from build123d import *

# Parameters (mm, degrees)
BOSS_EXTRUDE1_DEPTH                               = 12.7
FILLET1_R                                         = 12.7
F_1_4_0_25_DIAMETER_HOLE1_D                       = 6.35
HOLE1_D                                           = 3.175
HOLE1_DEPTH                                       = 38.1
HOLE1_CSINK_D                                     = 10.16
HOLE1_CSINK_ANGLE                                 = 82
HOLE1_TIP                                         = 0.9538662327062519
F_5_16_CLEARANCE_HOLE1_D                          = 8.72998
CUT_EXTRUDE1_DEPTH                                = 998.2767957894854
FILLET2_R                                         = 3.175
CSK_FOR_8_FLAT_HEAD_MACHINE_SCREW_100_D           = 4.9149
CSK_FOR_8_FLAT_HEAD_MACHINE_SCREW_100_DEPTH       = 22.225
CSK_FOR_8_FLAT_HEAD_MACHINE_SCREW_100_CSINK_D     = 16.0004506
CSK_FOR_8_FLAT_HEAD_MACHINE_SCREW_100_CSINK_ANGLE = 100
CSK_FOR_8_FLAT_HEAD_MACHINE_SCREW_100_TIP         = 1.476584928229278


with BuildPart() as part:
    # Sketch1 → Boss-Extrude1 (new body)
    with BuildSketch(Plane.XY):
        Polygon((-504.586893891522, 825.1654748045078), (-413.82187552728277, 548.4721148571872), (-471.5394528912339, 529.5387477161187), (-562.3044712554732, 806.2321076634394), align=None)
        Polygon((-421.80123191535296, 572.7968488683923), (-413.82187552728277, 548.4721148571872), (-401.754552912923, 552.4306151945574), (-409.7339093009929, 576.7553492057625), align=None)
        Polygon((-504.586893891522, 825.1654748045078), (-492.51957127716224, 829.123975141878), (-484.5402148890918, 804.7992411306724), (-496.6075375034517, 800.8407407933022), align=None)
    extrude(amount=BOSS_EXTRUDE1_DEPTH)

    # Fillet1
    fillet1_edges = [part.edges().sort_by_distance(p)[0] for p in [
        (-401.754552912923, 552.4306151945574, 6.35),
        (-471.5394528912339, 529.5387477161187, 6.35),
        (-562.3044712554732, 806.2321076634394, 6.35),
        (-492.51957127716224, 829.123975141878, 6.35),
    ]]
    fillet(fillet1_edges, radius=FILLET1_R)

    # 1/4 (0.25) Diameter Hole1 (through all)
    with Locations(Plane(origin=(0, 0, 0), x_dir=(-1, 0, 0), z_dir=(0, 0, -1))):
        with Locations((496.607537503, 800.840740793), (421.801231915, 572.796848868)):
            Hole(F_1_4_0_25_DIAMETER_HOLE1_D / 2)

    # Hole1
    with Locations(Plane(origin=(-72.82198225638447, -450.30656055117834, -91.0749999969487), x_dir=(-4.8e-16, -1.6e-16, -1), z_dir=(0.9501828830204595, 0.3116929399504066, 0))):
        with Locations((-97.424999997, 1099.959715498), (-97.424999997, 1301.859715498), (-97.424999997, 1200.909715498)):
            CounterSinkHole(HOLE1_D / 2, HOLE1_CSINK_D / 2, depth=HOLE1_DEPTH, counter_sink_angle=HOLE1_CSINK_ANGLE)
            with Locations((0, 0, -(HOLE1_DEPTH + HOLE1_TIP / 2))):  # 118° drill point
                Cone(0, HOLE1_D / 2, HOLE1_TIP, mode=Mode.SUBTRACT)

    # 5/16 Clearance Hole1 (through all)
    with Locations(Plane.XY.offset(12.7)):
        with Locations((-546.278648304, 798.123285386), (-500.628393554, 813.09815219), (-463.430630614, 545.564570668), (-417.780375865, 560.539437472), (-501.837808805, 672.833553111)):
            Hole(F_5_16_CLEARANCE_HOLE1_D / 2)

    # Sketch9 → Cut-Extrude1 (cut, through all)
    with BuildSketch(Plane.XY.offset(12.7)):
        with BuildLine():
            Line((-529.6953014924577, 821.9412393048426), (-514.6111482245083, 826.8893647265553))
            ThreePointArc((-514.6111482245083, 826.8893647265553), (-508.60146461760905, 823.8485563726845), (-511.6422729714802, 817.838872765785))
            Line((-511.6422729714802, 817.838872765785), (-526.72642623943, 812.8907473440726))
            ThreePointArc((-526.72642623943, 812.8907473440726), (-532.7361098463288, 815.9315556979438), (-529.6953014924577, 821.9412393048426))
        make_face()
        with BuildLine():
            Line((-546.3745591048678, 778.043051296225), (-518.8053014409139, 693.9993230871839))
            ThreePointArc((-518.8053014409139, 693.9993230871839), (-522.8597125794092, 685.9864116113188), (-530.8726240552741, 690.0408227498137))
            Line((-530.8726240552741, 690.0408227498137), (-558.4418817192275, 774.084550958855))
            ThreePointArc((-558.4418817192275, 774.084550958855), (-554.3874705807326, 782.0974624347199), (-546.3745591048678, 778.043051296225))
        make_face()
        with BuildLine():
            Line((-435.961407875191, 536.1973873967519), (-420.87725460724124, 541.1455128184643))
            ThreePointArc((-420.87725460724124, 541.1455128184643), (-417.83644625337, 547.1551964253636), (-423.8461298602691, 550.1960047792348))
            Line((-423.8461298602691, 550.1960047792348), (-438.93028312821866, 545.2478793575218))
            ThreePointArc((-438.93028312821866, 545.2478793575218), (-441.9710914820897, 539.2381957506229), (-435.961407875191, 536.1973873967519))
        make_face()
        with BuildLine():
            Line((-475.40204242747944, 561.6863044207033), (-502.9713000914331, 645.7300326297446))
            ThreePointArc((-502.9713000914331, 645.7300326297446), (-510.9842115672985, 649.7844437682393), (-515.038622705793, 641.7715322923741))
            Line((-515.038622705793, 641.7715322923741), (-487.4693650418391, 557.7278040833331))
            ThreePointArc((-487.4693650418391, 557.7278040833331), (-479.4564535659742, 553.6733929448383), (-475.40204242747944, 561.6863044207033))
        make_face()
    extrude(amount=-CUT_EXTRUDE1_DEPTH, mode=Mode.SUBTRACT)

    # Fillet2
    fillet2_edges = [part.edges().sort_by_distance(p)[0] for p in [
        (-417.83644625337, 547.1551964253636, 6.35),
        (-441.97109148208983, 539.2381957506232, 6.35),
        (-522.859712579409, 685.9864116113188, 6.35),
        (-554.3874705807328, 782.0974624347198, 6.35),
        (-510.9842115672983, 649.7844437682394, 6.35),
        (-479.45645356597436, 553.6733929448382, 6.35),
        (-508.60146461760894, 823.8485563726842, 6.35),
        (-532.7361098463288, 815.9315556979437, 6.35),
    ]]
    fillet(fillet2_edges, radius=FILLET2_R)

    # CSK for #8 Flat Head Machine Screw (100)2
    with Locations(Plane(origin=(322.2568407232823, -320.70700445811474, 0), x_dir=(-0.9977564584489056, 0.06694811142592035, 0), z_dir=(0, 0, -1))):
        with Locations((876.906978493, 992.672305446), (833.265235439, 884.655200952), (904.92137181, 1028.108129087), (833.558815764, 851.479604792)):
            CounterSinkHole(CSK_FOR_8_FLAT_HEAD_MACHINE_SCREW_100_D / 2, CSK_FOR_8_FLAT_HEAD_MACHINE_SCREW_100_CSINK_D / 2, depth=CSK_FOR_8_FLAT_HEAD_MACHINE_SCREW_100_DEPTH, counter_sink_angle=CSK_FOR_8_FLAT_HEAD_MACHINE_SCREW_100_CSINK_ANGLE)
            with Locations((0, 0, -(CSK_FOR_8_FLAT_HEAD_MACHINE_SCREW_100_DEPTH + CSK_FOR_8_FLAT_HEAD_MACHINE_SCREW_100_TIP / 2))):  # 118° drill point
                Cone(0, CSK_FOR_8_FLAT_HEAD_MACHINE_SCREW_100_D / 2, CSK_FOR_8_FLAT_HEAD_MACHINE_SCREW_100_TIP, mode=Mode.SUBTRACT)


solid = part.part
Build history of the part. All positions in model axes, mm. A direction names the side the tool comes from. Coordinates: 2 decimals unless noted, no trailing zeros. One line per question, with ' | ' between items. Start each with the question number.
Q1. Saw through at A-A (z = 2). Count the separate pieces of the cut face and the enclosed holes in it, then the cut area to 3 significant figures.
Q2. Two-plate mould, pull along X, no slides. Class faces 4 (the face through (-495.02, 824.492, 6.439)), 5 (the face through (-407.695, 570.541, 6.261)), 6 (the face through (-486.398, 731.167, 4.425)), 7 (the face through (-518.754, 690.205, 6.439)): +X half, -X half, draft (parallel to the pull), parting line (faces both ways), or undercut.
Q3. Flat gauge pins, fed straight in: pin 1 Ø4 at (x, y) = (-421.8, 572.8) entering from +Z; pin 2 Ø4 at (y, z) = (718.5, 9.5) entering from +X; pin 3 Ø1 at (x, z) = (-459, 7) entering from +Y; pin 4 Ø2 at (y, z) = (606, 4.5) entering from +X (3 decimals). Where does each tip first touch, or does it go through?
Q4. 3-axis set-ups, long thin cutter, end or side, ignore diameter. For faces 1 (the face through (-465.777, 549.245, 6.261)), 2 (the face through (-519.08, 815.4, 6.44)), 3 (the face through (-431.283, 547.757, 6.439)): which of +Z, -Z, +X, -X, +Y, -Y reach the whole face in a straight line?
Q5. Probe L1, parallel to Y at x = -511.5, z = 6; L2, parallel to X at y = 545, z = 6.25; L3, parallel to X at y = 767, z = 4.5. List the from-to ranges inside material, lowest first. Write a range as from..to.
Check values:
1) separate pieces: 1 | enclosed holes: 9 | area: 16,000 mm2
2) face 4: parting line | face 5: +X half | face 6: undercut | face 7: -X half
3) pin 1: passes through | pin 2: stops at x = -468.94 | pin 3: stops at y = 685.76 | pin 4: stops at x = -432.365
4) face 1: +Z, -Z | face 2: +Z, -Z, +Y | face 3: +Z, -Z, -Y
5) L1: y = 651.62..763.24, 768.12..774.28, 777.54..817.89 | L2: x = -476.61..-467.76, -459.1..-439.54 | L3: x = -542.75..-514.09, -509.52..-485.51
